Source: CAD feature listing. Evaluate the final solid. Frame: model axes, mm. Face numbers are marked on the shaded views. A direction names the side the tool comes from. Coordinates: 2 decimals unless noted, no trailing zeros. Order: outer loops, then holes, each group sorted by start corner. A loop starts at its lowest first (then second) coordinate and runs counter-clockwise, first axis right, second up.
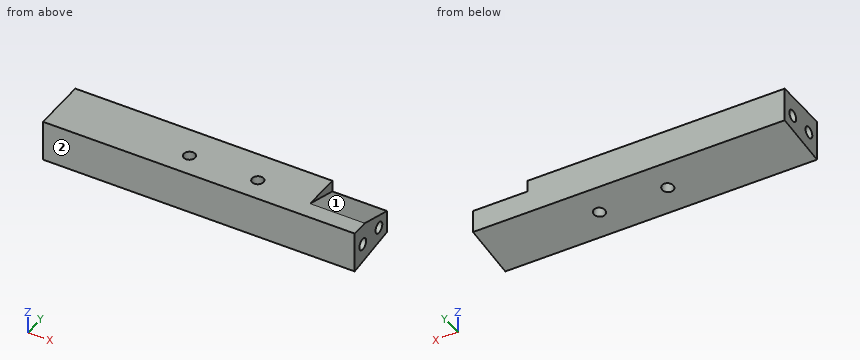
```python
from build123d import *

# Parameters (mm, degrees)
RESSALTO_EXTRUS_O1_DEPTH      = 68.4
CORTE_EXTRUS_O1_DEPTH         = 12
FURO_ROSCADO_DE_M3X0_51_D     = 2.5
FURO_ROSCADO_DE_M3X0_51_DEPTH = 8.5
FURO_ROSCADO_DE_M3X0_51_TIP   = 0.751075774
FURO_ROSCADO_DE_M3X0_52_D     = 2.5
FURO_ROSCADO_DE_M3X0_52_DEPTH = 8.5
FURO_ROSCADO_DE_M3X0_52_TIP   = 0.751075774
FURO_ROSCADO_DE_M3X0_53_D     = 2.5


with BuildPart() as part:
    # Esboço1 → Ressalto-extrusão1 (new body)
    with BuildSketch(Plane(origin=(0, 0, 0), x_dir=(0, 0, -1), z_dir=(1, 0, 0))):
        Polygon((-4.5, -6), (4.5, -6), (3.026585269, 6), (-4.5, 6), align=None)
    extrude(amount=RESSALTO_EXTRUS_O1_DEPTH)

    # Esboço2 → Corte-extrusão1 (cut)
    with BuildSketch(Plane(origin=(68.4, 0, 0), x_dir=(0, 0, -1), z_dir=(1, 0, 0))):
        Polygon((-1.973414731, 6), (-4.5, -2.264088043), (-4.5, 6), align=None)
    extrude(amount=-CORTE_EXTRUS_O1_DEPTH, mode=Mode.SUBTRACT)

    # Furo roscado de M3x0.51
    with Locations(Plane(origin=(68.4, 0, 0), x_dir=(0, 0, -1), z_dir=(1, 0, 0))):
        with Locations((0, -3), (0, 3)):
            Hole(FURO_ROSCADO_DE_M3X0_51_D / 2, depth=FURO_ROSCADO_DE_M3X0_51_DEPTH)
            with Locations((0, 0, -(FURO_ROSCADO_DE_M3X0_51_DEPTH + FURO_ROSCADO_DE_M3X0_51_TIP / 2))):  # 118° drill point
                Cone(0, FURO_ROSCADO_DE_M3X0_51_D / 2, FURO_ROSCADO_DE_M3X0_51_TIP, mode=Mode.SUBTRACT)

    # Furo roscado de M3x0.52
    with Locations(Plane.ZY):
        with Locations((0, 3), (0, -3)):
            Hole(FURO_ROSCADO_DE_M3X0_52_D / 2, depth=FURO_ROSCADO_DE_M3X0_52_DEPTH)
            with Locations((0, 0, -(FURO_ROSCADO_DE_M3X0_52_DEPTH + FURO_ROSCADO_DE_M3X0_52_TIP / 2))):  # 118° drill point
                Cone(0, FURO_ROSCADO_DE_M3X0_52_D / 2, FURO_ROSCADO_DE_M3X0_52_TIP, mode=Mode.SUBTRACT)

    # Furo roscado de M3x0.53 (through all)
    with Locations(Plane(origin=(0, 0.455211444, -3.707399697), x_dir=(-1, 0, 0), z_dir=(0, 0.121869343, -0.992546152))):
        with Locations((-29.2, -0.464432322), (-44.2, -0.464432322)):
            Hole(FURO_ROSCADO_DE_M3X0_53_D / 2)


solid = part.part
```
1. Section query C-C, the plane x = 36. Output: boundary loops of the cut face in (y, z).
2. Section query D-D, the plane z = 3.25. Count the separate pieces of the cut face and the enclosed holes in it, plus the area to 3 significant figures.
3. Access query for the marked faces 1 and 2. Directions: +Z, -Z, +X, -X, +Y, -Y. A direction counts if a zero-diameter tool reaches every point of the face in a straight line with its end or side. Return the directions, or none.
4. Contact query for flat-ended pins moving along their axis: P1, Ø1.5, axis at y = -3, z = 0, coming from the -X side; P2, Ø5, axis at y = -3, z = 0.5, coming from the +X side; P3, Ø2, axis at y = 3, z = 0, coming from the +X side; P4, Ø4, axis at x = 10, y = 3.5, coming from the -Z side. Output: stop coordinate, or through.
5. Material intervals for line 1 along Y through (x, z) = (5, 0); line 2 along X through (y, z) = (3, 0); line 3 along Z through (x, y) = (63.5, -3), sorted ascending.
6. Section query A-A, the plane x = 61.5. Output: boundary loops of the cut face in (y, z).
7. Section query B-B, the plane x = 44. Output: boundary loops of the cut face in (y, z).
Answer key:
1. outline: (-6, -4.5) - (6, -3.03) - (6, 4.5) - (-6, 4.5) - close
2. separate pieces: 1
2. enclosed holes: 2
2. area: 761 mm2
3. face 1: +Z, +X, +Y
3. face 2: +Z, -Z, +X, -X, -Y
4. P1: stops at x = 8.8
4. P2: stops at x = 68.4
4. P3: stops at x = 59.75
4. P4: stops at z = -3.58
5. line 1: y = -6 to -4.25, -1.75 to 1.75, 4.25 to 6
5. line 2: x = 9.25 to 59.15
5. line 3: z = -4.13 to -1.25, 1.25 to 4.5
6. outline: (-6, -4.5) - (6, -3.03) - (6, 1.97) - (-2.26, 4.5) - (-6, 4.5) - close; hole circle Ø2.5 at (-3, 0); hole circle Ø2.5 at (3, 0)
7. outline: (-6, -4.5) - (-1.23, -3.91) - (-2.26, 4.5) - (-6, 4.5) - close; (0.22, 4.5) - (1.22, -3.61) - (6, -3.03) - (6, 4.5) - close
